Autodesk Inventor part; units mm, degrees
ref_plane "HG1_XY" through (0, 0, 0) normal (1, 0, 0) x (0, 0, -1)
ref_plane "HG1_YZ" through (0, 0, 0) normal (0, 0, -1) x (0, 1, 0)
ref_plane "HG1_ZX" through (0, 0, 0) normal (0, 1, 0) x (1, 0, 0)
sketch "Skizze_4" plane through (0, 0, 0) normal (1, 0, 0) x (0, 1, 0)
  line L0 (14.3, 31.7) -> (11.8, 31.7)
  arc A0 (11.8, 31.7) -> (6.3, 26.2) centre (11.8, 26.2) ccw
  line L1 (6.3, 26.2) -> (6.3, 23)
  arc A1 (0, 16.7) -> (6.3, 23) centre (0, 23) ccw
  arc A2 (0, 16.7) -> (-3.0486, 10.1104) centre (0, 12.7) ccw
  arc A3 (-2.8546, 2.1934) -> (-3.0486, 10.1104) centre (-7.8502, 6.0319) ccw
  arc A4 (-2.8546, 2.1934) -> (3.5986, 0.1012) centre (0, 0) ccw
  arc A5 (7.1983, 10.6002) -> (3.5986, 0.1012) centre (19.3921, 0.5528) ccw
  arc A6 (7.1983, 10.6002) -> (11.8856, 24.4701) centre (-8.7, 23.7) ccw
  arc A7 (12.685, 25.3) -> (11.8856, 24.4701) centre (12.685, 24.5) ccw
  line L2 (12.685, 25.3) -> (14.3, 25.3)
  line L3 (14.3, 25.3) -> (14.3, 31.7)
  circle A8 centre (5.8, 12.7) radius 0.965
extrude "Extrusion1" add sketch "Skizze_4" along normal mid plane 4
sketch "Sketch_1" plane through (0, 0, 0) normal (1, 0, 0) x (0, 1, 0)
  line L0 (14.3, 32.7) -> (11.8, 32.7)
  arc A0 (11.8, 32.7) -> (5.3, 26.2) centre (11.8, 26.2) ccw
  line L1 (5.3, 26.2) -> (5.3, 23)
  arc A1 (4.9518, 21.1105) -> (5.3, 23) centre (0, 23) ccw
  arc A2 (4.9518, 21.1105) -> (5.1789, 20.0469) centre (5.8861, 20.754) ccw
  line L2 (5.1789, 20.0469) -> (9.6942, 15.5317)
  arc A3 (9.6942, 15.5317) -> (11.3334, 15.8766) centre (10.4013, 16.2388) ccw
  arc A4 (11.3334, 15.8766) -> (12.7966, 23.3177) centre (-8.8, 23.7) ccw
  arc A5 (13.7965, 24.3) -> (12.7966, 23.3177) centre (13.7965, 23.3) ccw
  line L3 (13.7965, 24.3) -> (14.3, 24.3)
  arc A6 (14.3, 24.3) -> (15.3, 25.3) centre (14.3, 25.3) ccw
  line L4 (15.3, 25.3) -> (15.3, 31.7)
  arc A7 (15.3, 31.7) -> (14.3, 32.7) centre (14.3, 31.7) ccw
extrude "Extrusion2" add sketch "Sketch_1" along normal mid plane 6
sketch "Skizze_5_ALT_Drilling_1" plane through (0, 0, 0) normal (0, 1, 0) x (-1, 0, 0)
  line L0 (10, 0) -> (-10, 0)
  line L1 (-10, 0) -> (-10, 1.6)
  line L2 (-10, 1.6) -> (10, 1.6)
  line L3 (10, 1.6) -> (10, 0)
  line L4 (10, 0) -> (-10, 0)
revolve "Revolution1" cut sketch "Skizze_5_ALT_Drilling_1" angle 360 about axis through (-10, 0, 0) along (-1, 0, 0)
sketch "Skizze_6_ALT_Drilling_2" plane through (0, 0, 0) normal (0, 1, 0) x (-1, 0, 0)
  line L0 (10, 12.7) -> (-10, 12.7)
  line L1 (-10, 12.7) -> (-10, 14.3)
  line L2 (-10, 14.3) -> (10, 14.3)
  line L3 (10, 14.3) -> (10, 12.7)
  line L4 (10, 12.7) -> (-10, 12.7)
revolve "Revolution2" cut sketch "Skizze_6_ALT_Drilling_2" angle 360 about axis through (-10, 0, 12.7) along (-1, 0, 0)
sketch "Sketch_2" plane through (0, 16.4, 0) normal (0, 1, 0) x (1, 0, 0)
  arc A0 (-9.5, -24.3) -> (-9.5, -32.7) centre (-9.5, -28.5) ccw
  line L0 (-9.5, -32.7) -> (9.5, -32.7)
  arc A1 (9.5, -32.7) -> (9.5, -24.3) centre (9.5, -28.5) ccw
  line L1 (9.5, -24.3) -> (-9.5, -24.3)
extrude "Extrusion3" add sketch "Sketch_2" against normal blind 6.1
sketch "Sketch_3" plane through (0, 0, 0) normal (1, 0, 0) x (0, 1, 0)
  line L0 (-12.0571, 36.1801) -> (-12.0571, -15.6384)
  line L1 (-12.0571, -15.6384) -> (20.4908, -15.6384)
  line L2 (20.4908, -15.6384) -> (20.4908, 36.1801)
  line L3 (20.4908, 36.1801) -> (-12.0571, 36.1801)
  line L4 (15.4, 32.7) -> (11.8, 32.7)
  arc A0 (11.8, 32.7) -> (5.3, 26.2) centre (11.8, 26.2) ccw
  line L5 (5.3, 26.2) -> (-6.4975, 26.2)
  line L6 (-6.4975, 26.2) -> (-6.4975, -9.3)
  line L7 (-6.4975, -9.3) -> (15.4, -9.3)
  line L8 (15.4, -9.3) -> (15.4, 24.3)
  arc A1 (15.4, 24.3) -> (16.4, 25.3) centre (15.4, 25.3) ccw
  line L9 (16.4, 25.3) -> (16.4, 31.7)
  arc A2 (16.4, 31.7) -> (15.4, 32.7) centre (15.4, 31.7) ccw
extrude "Extrusion4" cut sketch "Sketch_3" along normal mid plane 40
sketch "Sketch_4" plane through (0, 0, 32.7) normal (0, 0, 1) x (1, 0, 0)
  line L0 (-22.6525, -16.2217) -> (-3, -16.2217)
  line L1 (-3, -16.2217) -> (-3, 10.3)
  arc A0 (-3, 10.3) -> (-4, 11.3) centre (-4, 10.3) ccw
  line L2 (-4, 11.3) -> (-12.7, 11.3)
  arc A1 (-13.7, 12.3) -> (-12.7, 11.3) centre (-12.7, 12.3) ccw
  line L3 (-13.7, 12.3) -> (-13.7, 15.4)
  arc A2 (-12.7, 16.4) -> (-13.7, 15.4) centre (-12.7, 15.4) ccw
  line L4 (-12.7, 16.4) -> (-2.7982, 16.4)
  arc A3 (-0.583, 15.6875) -> (-2.7982, 16.4) centre (-2.7982, 12.6) ccw
  arc A4 (-0.583, 15.6875) -> (0.583, 15.6875) centre (0, 16.5) ccw
  arc A5 (2.7982, 16.4) -> (0.583, 15.6875) centre (2.7982, 12.6) ccw
  line L5 (2.7982, 16.4) -> (12.7, 16.4)
  arc A6 (13.7, 15.4) -> (12.7, 16.4) centre (12.7, 15.4) ccw
  line L6 (13.7, 15.4) -> (13.7, 12.3)
  arc A7 (12.7, 11.3) -> (13.7, 12.3) centre (12.7, 12.3) ccw
  line L7 (12.7, 11.3) -> (4, 11.3)
  arc A8 (4, 11.3) -> (3, 10.3) centre (4, 10.3) ccw
  line L8 (3, 10.3) -> (3, -16.2217)
  line L9 (3, -16.2217) -> (21.2638, -16.2217)
  line L10 (21.2638, -16.2217) -> (21.2638, 23.8758)
  line L11 (21.2638, 23.8758) -> (-22.6525, 23.8758)
  line L12 (-22.6525, 23.8758) -> (-22.6525, -16.2217)
extrude "Extrusion5" cut sketch "Sketch_4" against normal blind 10
ref_plane "HG1_XY" through (0, 0, 0) normal (1, 0, 0) x (0, 0, -1)
ref_plane "HG1_YZ" through (0, 0, 0) normal (0, 0, -1) x (0, 1, 0)
ref_plane "HG1_ZX" through (0, 0, 0) normal (0, 1, 0) x (1, 0, 0)
ref_plane "HG2_XY" through (0, 0, 12.7) normal (1, 0, 0) x (0, 0, -1)
ref_plane "HG2_YZ" through (0, 0, 12.7) normal (0, 0, -1) x (0, 1, 0)
ref_plane "HG2_ZX" through (0, 0, 12.7) normal (0, 1, 0) x (1, 0, 0)
ref_plane "HG3_XY" through (0, 0, 0) normal (0, 0, 1) x (1, 0, 0)
ref_plane "HG3_YZ" through (0, 0, 0) normal (1, 0, 0) x (0, 1, 0)
ref_plane "HG3_ZX" through (0, 0, 0) normal (0, 1, 0) x (0, 0, 1)
properties part number "305104_105"
Input: part model. Units: mm. Frame: model coordinates. A direction names the side the tool comes from. Coordinates: 2 decimals unless noted, no trailing zeros. Loops run counter-clockwise (first coordinate to the right, second up) from the corner with the lowest first, then second, coordinate; pieces in that order, holes last.
(1) Pull-direction query (Y, two-part tool) for faces 4 (the face through (-3, 9, 24)), 5 (the face through (2.545, 16.099, 32.415)), 6 (the face through (-0.028, 0.481, 14.226)), 7 (the face through (-0.78, 7.46, 31.04)); classes: released by +Y, released by -Y, zero draft, split by the parting line, or undercut.
(2) Material intervals for probe 1 along Y at (x, z) = (-0.95, 0); probe 2 along X at (y, z) = (3, 15); probe 3 along X at (y, z) = (6, 20), sorted ascending.
(3) Section B-B on z = 28.5. Return the cut outline in (x, y), then the cut area to 3 significant figures.
(4) Section A-A on x = -6.5. Return the cut outline in (y, z).
(5) Section C-C on y = 15. Return the cut outline in (x, z).
(6) First-contact query: pin 1 Ø2.5 at (y, z) = (9, 23.5) entering from -X; pin 2 Ø2 at (y, z) = (1.5, 10.5) entering from -X; pin 3 Ø1.6 at (x, z) = (0, 25.5) entering from -Y. Flat tips, straight axial feed; report the tip coordinate or a pass-through.
(7) Set-up query: faces 1 (the face through (-2.709, 6.903, 18.323)), 2 (the face through (0, 5.3, 25)), 3 (the face through (-8, 11.3, 29)). Return all of +Z, -Z, +X, -X, +Y, -Y with unobstructed straight access to the full face (end or side cutting, diameter ignored); none if empty.
(8) Section D-D on x = -1.5. Count the separate pieces of the cut face and the enclosed holes in it, then the cut area to 3 significant figures.
Data:
1. face 4: zero draft
1. face 5: released by +Y
1. face 6: undercut
1. face 7: released by -Y
2. probe 1: y = -3.6 to -1.6, 1.6 to 3.6
2. probe 2: x = -2 to 2
2. probe 3: x = -3 to 3
3. outline: (-13.7, 12.3) arc R1 ccw to (-12.7, 11.3) - (-4, 11.3) arc R1 cw to (-3, 10.3) - (-3, 5.72) - (3, 5.72) - (3, 10.3) arc R1 cw to (4, 11.3) - (12.7, 11.3) arc R1 ccw to (13.7, 12.3) - (13.7, 15.4) arc R1 ccw to (12.7, 16.4) - (2.8, 16.4) arc R3.8 ccw to (0.58, 15.69) arc R1 cw to (-0.58, 15.69) arc R3.8 ccw to (-2.8, 16.4) - (-12.7, 16.4) arc R1 ccw to (-13.7, 15.4) - close
3. area: 171 mm2
4. outline: (11.3, 24.3) - (15.4, 24.3) arc R1 ccw to (16.4, 25.3) - (16.4, 31.7) arc R1 ccw to (15.4, 32.7) - (11.8, 32.7) arc R6.5 ccw to (11.3, 32.68) - close
5. outline: (-9.5, 24.3) - (9.5, 24.3) arc R4.2 ccw to (9.5, 32.7) - (-9.5, 32.7) arc R4.2 ccw to start
6. pin 1: stops at x = -3
6. pin 2: stops at x = -2
6. pin 3: stops at y = 5.3
7. face 1: -Y
7. face 2: +Z, +X, -X, -Y
7. face 3: +Z, -Z, -X, -Y
8. separate pieces: 1
8. enclosed holes: 3
8. area: 295 mm2
